For this review, take the finished solid that the model builds, in its own axes (mm). A direction names the side the tool comes from. Round coordinates to 2 decimals unless told otherwise and drop trailing zeros. Order: outer loops, then holes, each group sorted by start corner. A loop starts at its lowest first (then second) coordinate and runs counter-clockwise, first axis right, second up.
Autodesk Inventor part; units mm, degrees
ref_plane "YZ Plane" through (0, 0, 0) normal (1, 0, 0) x (0, 1, 0)
ref_plane "XZ Plane" through (0, 0, 0) normal (0, 1, 0) x (-1, 0, 0)
ref_plane "XY Plane" through (0, 0, 0) normal (0, 0, 1) x (1, 0, 0)
sketch "Sketch1" plane through (0, 0, 0) normal (0, 0, 1) x (1, 0, 0)
  line L0 (0, 0) -> (8.5363, 0)
  circle A0 centre (0, 9) radius 1.5
  circle A1 centre (0, -9) radius 1.5
  line L1 (-4.7525, 12.0011) -> (4.7525, 12.0011)
  line L2 (4.7525, 12.0011) -> (4.7525, -12.0011)
  line L3 (4.7525, -12.0011) -> (-4.7525, -12.0011)
  line L4 (-4.7525, -12.0011) -> (-4.7525, 12.0011)
  ellipse E0 centre (0, 0) end of major axis (0, 6.027) minor radius 4.3359
  ellipse E1 centre (-34.059, -8.6397) end of major axis (-34.059, -4.9131) minor radius 2.5528
  ellipse E2 centre (-34.1113, -8.6921) end of major axis (-34.1113, -2.6651) minor radius 4.3359
  point P0 (0, 12.0011)
  point P1 (0, -12.0011)
  point P2 (-4.7525, 0)
  point P3 (4.7525, 0)
extrude "Extrusion1" add sketch "Sketch1" along normal blind 5 contours L2 L3 L4 L1
sketch "Sketch2" plane through (0, 0, 5) normal (0, 0, 1) x (1, 0, 0)
  point P0 (0, 0)
sketch "Sketch3" plane through (0, 0, 5) normal (0, 0, 1) x (1, 0, 0)
  ellipse E0 centre (0, 0) end of major axis (0, -6.027) minor radius 4.3359
extrude "Extrusion2" add sketch "Sketch3" along normal blind 50 and the other way blind 5
chamfer "Chamfer1" distance 2 angle 45 1 edges at (0, 6.027, 55)
fillet "Fillet1" radius 1 1 edges at (0, 12.0011, 5)
fillet "Fillet2" radius 1 1 edges at (0, -12.0011, 5)
properties part number "apoioP"
Q1. Tool access review of faces 1 (the face through (-4, 3, 5)), 2 (the face through (-4.752, 0, 2)): name each direction out of +Z, -Z, +X, -X, +Y, -Y from which nothing blocks a thin tool from reaching the whole face with its end or side.
Q2. Wall thickness on line 1 (Y direction, x = 0, z = 1.3); line 2 (Z direction, x = 4.25, y = 4.5); line 3 (Y direction, x = 0, z = 44): over which ranges is each line inside the solid? List them lowest first.
Q3. Take a section at B-B, the plane x = 0. Count the separate pieces of the cut face and the enclosed holes in it, plus the area to 3 significant figures.
Q4. Take a section at A-A, the plane y = 9. State the section outline as (x, z) points.
Q5. Clearance check with flat-ended pins moving along their axes: pin 1 (3 mm diameter, centred on x = 3.5, z = 29, fed in from +Y); pin 2 (3 mm diameter, centred on x = 0, z = 29, fed in from +Y); pin 3 (3.5 mm diameter, centred on x = 0, y = -9, fed in from +Z). State where each tip first meets the part, or that it passes through.
Working result:
1. face 1: +Z
1. face 2: +Z, -Z, -X, +Y, -Y
2. line 1: y = -12 to -10.5, -7.5 to 7.5, 10.5 to 12
2. line 2: z = 0 to 5
2. line 3: y = -6.03 to 6.03
3. separate pieces: 3
3. enclosed holes: 0
3. area: 688 mm2
4. outline: (-4.75, 0) - (-1.5, 0) - (-1.5, 5) - (-4.75, 5) - close; (1.5, 0) - (4.75, 0) - (4.75, 5) - (1.5, 5) - close
5. pin 1: stops at y = 5.35
5. pin 2: stops at y = 6.03
5. pin 3: stops at z = 5
